Here's how the part is built. I have some questions about the finished solid (model axes, mm). Face numbers are marked on the shaded views. Round coordinates to 2 decimals unless told otherwise and drop trailing zeros. Loops run counter-clockwise (first coordinate to the right, second up) from the corner with the lowest first, then second, coordinate; pieces in that order, holes last. Notation, with made-up numbers: (54, 23) - (86, 23) arc R20 cw to (86, 35) - close; hole circle Ø5 at (51, 13.25). An arc over 180 degrees is marked (long way). Answer as a JSON object with one key per item and string values. Group by question number.
1) I want a section at D-D, the plane z = 13.75. Please give me the cut outline in (x, y).
2) I want a section at A-A, the plane y = 0. Please give me the cut outline in (x, z), then the cut area to 3 significant figures.
3) Will these pins go through, and if not, where does the flat tip stop? P1, Ø5.5, axis at x = -12.7, y = 12.7, coming from the -Z side; P2, Ø1.2, axis at x = -10.39, y = 6, coming from the -Z side.
4) I want a section at C-C, the plane x = 8. Please give me the cut outline in (y, z).
5) If we mould it in two halves opening along X, with no side actions, what happens to the marked faces 1, 2, 3 and 4? For each: pulls with the +X half, pulls with the -X half, needs draft (parallel to the pull), parting line crosses it, or undercut.
6) I want a section at B-B, the plane z = 4.75. Please give me the cut outline in (x, y).
7) If I drill on line 1 along X through (y, z) = (12.7, 13.15); line 2 along X through (y, z) = (-12, 4.6), over which ranges is the centre line in solid material (lowest first)? Write a range as [from, to].
from build123d import *

# Parameters (mm, degrees)
F0_R     = 10.1
F1_DEPTH = 16
F3_D     = 3.5
F3_DEPTH = 6
F3_TIP   = 1.0515060833
F5_D     = 2
F5_DEPTH = 6
F5_TIP   = 0.600860619


with BuildPart() as f1:
    # F0 (on Top) → F1 (new body)
    with BuildSketch(Plane.XY):
        with BuildLine():
            Line((-15.5, -17.5), (15.5, -17.5))
            ThreePointArc((15.5, -17.5), (16.9142135624, -16.9142135624), (17.5, -15.5))
            Line((17.5, -15.5), (17.5, 15.5))
            ThreePointArc((17.5, 15.5), (16.9142135624, 16.9142135624), (15.5, 17.5))
            Line((15.5, 17.5), (-15.5, 17.5))
            ThreePointArc((-15.5, 17.5), (-16.9142135624, 16.9142135624), (-17.5, 15.5))
            Line((-17.5, 15.5), (-17.5, -15.5))
            ThreePointArc((-17.5, -15.5), (-16.9142135624, -16.9142135624), (-15.5, -17.5))
        make_face()
        Circle(F0_R, mode=Mode.SUBTRACT)
    extrude(amount=F1_DEPTH)

    # F3
    with Locations(Plane.XY.offset(16)):
        with Locations((-12.7, 12.7), (12.7, 12.7), (12.7, -12.7), (-12.7, -12.7)):
            Hole(F3_D / 2, depth=F3_DEPTH)
            with Locations((0, 0, -(F3_DEPTH + F3_TIP / 2))):  # 118° drill point
                Cone(0, F3_D / 2, F3_TIP, mode=Mode.SUBTRACT)

    # F5
    with Locations(Plane(origin=(0, 0, 0), x_dir=(1, 0, 0), z_dir=(0, 0, -1))):
        with Locations((0, 12), (10.3923048454, -6), (-10.3923048454, -6)):
            Hole(F5_D / 2, depth=F5_DEPTH)
            with Locations((0, 0, -(F5_DEPTH + F5_TIP / 2))):  # 118° drill point
                Cone(0, F5_D / 2, F5_TIP, mode=Mode.SUBTRACT)


solid = f1.part
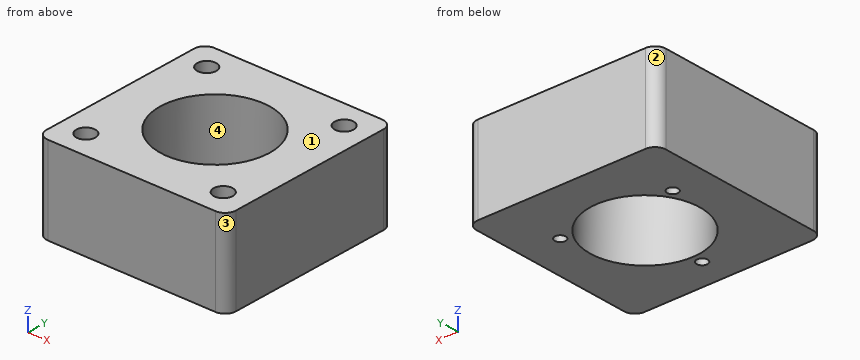
Outcome:
{
 "1": {"outline": "(-17.5, -15.5) arc R2 ccw to (-15.5, -17.5) - (15.5, -17.5) arc R2 ccw to (17.5, -15.5) - (17.5, 15.5) arc R2 ccw to (15.5, 17.5) - (-15.5, 17.5) arc R2 ccw to (-17.5, 15.5) - close; hole circle Ø3.5 at (-12.7, -12.7); hole circle Ø3.5 at (-12.7, 12.7); hole circle Ø20.2 at (0, 0); hole circle Ø3.5 at (12.7, -12.7); hole circle Ø3.5 at (12.7, 12.7)"},
 "2": {"outline": "(-17.5, 0) - (-10.1, 0) - (-10.1, 16) - (-17.5, 16) - close; (10.1, 0) - (17.5, 0) - (17.5, 16) - (10.1, 16) - close", "area": "237 mm^2"},
 "3": {"P1": "z = 0", "P2": "z = 6.24"},
 "4": {"outline": "(-17.5, 0) - (-6.17, 0) - (-6.17, 16) - (-17.5, 16) - close; (6.17, 0) - (17.5, 0) - (17.5, 16) - (6.17, 16) - close"},
 "5": {"face 1": "needs draft", "face 2": "pulls with the -X half", "face 3": "pulls with the +X half", "face 4": "undercut"},
 "6": {"outline": "(-17.5, -15.5) arc R2 ccw to (-15.5, -17.5) - (15.5, -17.5) arc R2 ccw to (17.5, -15.5) - (17.5, 15.5) arc R2 ccw to (15.5, 17.5) - (-15.5, 17.5) arc R2 ccw to (-17.5, 15.5) - close; hole circle Ø2 at (-10.39, 6); hole circle Ø20.2 at (0, 0); hole circle Ø2 at (0, -12); hole circle Ø2 at (10.39, 6)"},
 "7": {"line 1": "[-17.5, -14.45], [-10.95, 10.95], [14.45, 17.5]", "line 2": "[-17.5, -1], [1, 17.5]"}
}
